The model under review builds one solid part; all positions refer to its coordinate system, in mm. A direction names the side the tool comes from. Coordinates: 2 decimals unless noted, no trailing zeros. Order: outer loops, then holes, each group sorted by start corner. A loop starts at its lowest first (then second) coordinate and runs counter-clockwise, first axis right, second up. Notation, with made-up numbers: M 26.5,-6 L 59.5,-6 A15 cw 59.5,-2 Z; hole C 61,-14 d10. An arc over 180 degrees is marked long. Write each question's results on one line, items separated by ' | '.
from build123d import *

# Parameters (mm, degrees)
SKETCH1_R           = 75
BOSS_EXTRUDE1_DEPTH = 20
SKETCH2_R           = 22.5
BOSS_EXTRUDE2_DEPTH = 780


with BuildPart() as part:
    # Sketch1 → Boss-Extrude1 (new body)
    with BuildSketch(Plane(origin=(0, 0, 0), x_dir=(1, 0, 0), z_dir=(0, 1, 0))):
        Circle(SKETCH1_R)
    extrude(amount=BOSS_EXTRUDE1_DEPTH)

    # Sketch2 → Boss-Extrude2 (add)
    with BuildSketch(Plane(origin=(0, 20, 0), x_dir=(1, 0, 0), z_dir=(0, 1, 0))):
        Circle(SKETCH2_R)
    extrude(amount=BOSS_EXTRUDE2_DEPTH)

    # Sketch4 → Cut-Revolve1 (revolve, cut)
    with BuildSketch(Plane(origin=(0, 0, 0), x_dir=(0, 0, -1), z_dir=(1, 0, 0))):
        with BuildLine():
            Line((0, 800), (-22.5, 800))
            ThreePointArc((-22.5, 800), (-12.311072252, 792.612587432), (0, 790))
            Line((0, 790), (0, 800))
        make_face()
    revolve(axis=Axis((0, 783.697468949, 0), (0, 1, 0)), mode=Mode.SUBTRACT)


solid = part.part
1) For faces 1 (the flat face through (-1, 0, -1)), 2 (the flat face through (16, 20, -18)), list the 3-axis set-ups (+Z, -Z, +X, -X, +Y, -Y) from which the entire face can be reached by the end or side of a thin tool; tool diameter is ignored.
Solutions:
face 1: +Z, -Z, +X, -X, -Y | face 2: +Y
2) Take a section at C-C on y = 692. State the section outline as (x, z) points, plus the area to 3 significant figures.
Solutions:
outline: C 0,0 d45 | area: 1,590 mm2
3) To check wall thickness, follow line 1 along Y through (x, z) = (-2, -0.5); line 2 along Y through (x, z) = (63, 7); line 3 along X through (y, z) = (171, -2). State the ranges of each line that lie inside material, in increasing order.
Solutions:
line 1: 0 to 790.07 | line 2: 0 to 20 | line 3: -22.41 to 22.41
4) For pin 1 (1.5 mm diameter, centred on x = 17, z = -27, fed in from +Y); pin 2 (1 mm diameter, centred on y = 511, z = 0, fed in from +X); pin 3 (6 mm diameter, centred on x = 13, y = 94.5, fed in from -Z), all flat-tipped, find the tip position at first contact; note any pin that passes through.
Solutions:
pin 1: y = 20 | pin 2: x = 22.5 | pin 3: z = -20.16
5) Take a section at D-D on x = -65. State the section outline as (y, z) points, plus the area to 3 significant figures.
Solutions:
outline: M 0,-37.42 L 20,-37.42 L 20,37.42 L 0,37.42 Z | area: 1,500 mm2
6) Take a section at B-B on x = 0. State the section outline as (y, z) points (1 decimal).
Solutions:
outline: M 0,-75 L 20,-75 L 20,-22.5 L 800,-22.5 A30.3 cw 800,22.5 L 20,22.5 L 20,75 L 0,75 Z
7) Take a section at A-A on z = 0. State the section outline as (x, y) points (1 decimal), plus the area to 3 significant figures.
Solutions:
outline: M -75,0 L 75,0 L 75,20 L 22.5,20 L 22.5,800 A30.3 cw -22.5,800 L -22.5,20 L -75,20 Z | area: 37,800 mm2
